```python
from build123d import *

# Parameters (mm, degrees)
F0_W     = 140
F0_H     = 140
F1_DEPTH = 140
F2_W     = 60
F2_H     = 130
F4_DEPTH = 130
F3_W     = 60
F3_H     = 130
F5_DEPTH = 130


with BuildPart() as f1:
    # F0 (on Top) → F1 (new body)
    with BuildSketch(Plane.XY):
        Rectangle(F0_W, F0_H)
    extrude(amount=F1_DEPTH)

    # F2 (on face) → F4 (cut)
    with BuildSketch(Plane.XY.offset(140)):
        with Locations((36.825541, 0.010989)):
            Rectangle(F2_W, F2_H)
    extrude(amount=-F4_DEPTH, mode=Mode.SUBTRACT)

    # F3 (on face) → F5 (cut)
    with BuildSketch(Plane.XY.offset(140)):
        with Locations((-36.683903, 1.187629)):
            Rectangle(F3_W, F3_H)
    extrude(amount=-F5_DEPTH, mode=Mode.SUBTRACT)


solid = f1.part
```
Source: CAD feature listing. Evaluate the final solid. Frame: model axes, mm. A direction names the side the tool comes from. Coordinates: 2 decimals unless noted, no trailing zeros. Order: outer loops, then holes, each group sorted by start corner. A loop starts at its lowest first (then second) coordinate and runs counter-clockwise, first axis right, second up. Notation, with made-up numbers: (42, -1.5) - (62, -1.5) arc R22 cw to (62, 31.5) - close; hole circle Ø2 at (0, 82). An arc over 180 degrees is marked (long way). One line per item, written item: value.
1) Reachability of faces 1 (the face through (-1, 70, 69)), 2 (the face through (36, 1, 10)) from +Z, -Z, +X, -X, +Y, -Y: full face, straight path, thin tool, end or side. Return the list, or none.
Computed values:
face 1: +Z, -Z, +X, -X, +Y
face 2: +Z
2) Mould query, pull axis X, two halves, no side actions, for faces 3 (the face through (-70, -1, 69)), 4 (the face through (36, 65.011, 76)), 5 (the face through (-1, 1, 0)), 6 (the face through (70, -1, 69)). Classes: released by +X, released by -X, zero draft, split by the parting line, or undercut.
Computed values:
face 3: released by -X
face 4: undercut
face 5: zero draft
face 6: released by +X
3) Cut plane C-C on y = -30.5. Output: boundary loops of the cut face in (x, z), plus the area to 3 significant figures.
Computed values:
outline: (-70, 0) - (70, 0) - (70, 140) - (66.83, 140) - (66.83, 10) - (6.83, 10) - (6.83, 140) - (-6.68, 140) - (-6.68, 10) - (-66.68, 10) - (-66.68, 140) - (-70, 140) - close
area: 4,000 mm^2
4) Contact query for a flat-ended pin moving along its axis: pin 1 (6 mm diameter, centred on x = 24, y = 1.5, fed in from +Z). Output: stop coordinate, or through.
Computed values:
pin 1: stops at z = 10
5) Cut plane B-B on x = -20. Output: boundary loops of the cut face in (y, z).
Computed values:
outline: (-70, 0) - (70, 0) - (70, 140) - (66.19, 140) - (66.19, 10) - (-63.81, 10) - (-63.81, 140) - (-70, 140) - close
6) Ray query, line 1 (X direction, y = 1, z = 101); line 2 (Y direction, x = 56, z = 30); line 3 (Y direction, x = -30.5, z = 21.5). Return the intervals inside material, ascending. Write a range as [from, to].
Computed values:
line 1: x = [-70, -66.68], [-6.68, 6.83], [66.83, 70]
line 2: y = [-70, -64.99], [65.01, 70]
line 3: y = [-70, -63.81], [66.19, 70]
7) Cut plane A-A on z = 84. Output: boundary loops of the cut face in (x, y), plus the area to 3 significant figures.
Computed values:
outline: (-70, -70) - (70, -70) - (70, 70) - (-70, 70) - close; hole (-66.68, -63.81) - (-6.68, -63.81) - (-6.68, 66.19) - (-66.68, 66.19) - close; hole (6.83, -64.99) - (66.83, -64.99) - (66.83, 65.01) - (6.83, 65.01) - close
area: 4,000 mm^2
